The listing builds one solid part. Answer for the finished solid, in the listing's coordinates (mm). A direction names the side the tool comes from. Give positions to 0.01 mm unless a question says otherwise; leave off trailing zeros. Write each loop counter-clockwise with the first axis right and the second up, starting at its lowest first coordinate (ties: lowest second). Pieces come first, ordered by that corner, then holes.
```python
from build123d import *

# Parameters (mm, degrees)
FILLET_1_R               = 2
CHAMFER_1_SIZE           = 2
CHAMFER_2_SIZE           = 0.5
SKETCH_4_R               = 15
CUT_EXTRUDE_3_DEPTH      = 20
CHAMFER_3_SIZE           = 3
CUT_EXTRUDE_4_DEPTH      = 161.780129369
CUT_EXTRUDE_4_DEPTH_BACK = 161.780129369
SKETCH_5_R               = 5.7226
CUT_EXTRUDE_5_DEPTH      = 14.5
CUT_EXTRUDE_6_DEPTH      = 161.780129369
CUT_EXTRUDE_6_DEPTH_BACK = 161.780129369
SKETCH_7_R               = 9
SKETCH_7_R_2             = 7


with BuildPart() as part:
    # ｽｹｯﾁ1 → 回転1 (revolve)
    with BuildSketch(Plane.XY, mode=Mode.PRIVATE) as revolve_1_sk:
        Polygon((0, 0), (0, 32.5), (81, 32.5), (81, 87), (100.5, 87), (100.5, 21), (103.5, 21), (103.5, 0), align=None)
    revolve(revolve_1_sk.sketch.rotate(Axis((0, 0, 0), (1, 0, 0)), 90), axis=Axis((0, 0, 0), (1, 0, 0)))

    # ﾌｨﾚｯﾄ1
    fillet_1_edges = [part.edges().sort_by_distance(p)[0] for p in [
        (81, 0, -32.5),
    ]]
    fillet(fillet_1_edges, radius=FILLET_1_R)

    # 面取り1
    chamfer_1_edges = [part.edges().sort_by_distance(p)[0] for p in [
        (0, 0, -32.5),
    ]]
    chamfer(chamfer_1_edges, length=CHAMFER_1_SIZE)

    # 面取り2
    chamfer_2_edges = [part.edges().sort_by_distance(p)[0] for p in [
        (103.5, 0, -21),
    ]]
    chamfer(chamfer_2_edges, length=CHAMFER_2_SIZE)

    # ｽｹｯﾁ4 → ｶｯﾄ - 押し出し3 (cut)
    with BuildSketch(Plane(origin=(0, 0, 0), x_dir=(0, 0, -1), z_dir=(1, 0, 0))):
        Circle(SKETCH_4_R)
    extrude(amount=CUT_EXTRUDE_3_DEPTH, mode=Mode.SUBTRACT)

    # 面取り3
    chamfer_3_edges = [part.edges().sort_by_distance(p)[0] for p in [
        (0, 0, 15),
    ]]
    chamfer(chamfer_3_edges, length=CHAMFER_3_SIZE)

    # ｽｹｯﾁ5 → ｶｯﾄ - 押し出し4 (cut, two sides: drawn at the far end of the back side and taken through both)
    with BuildSketch(Plane(origin=(0, 0, 0), x_dir=(0, 0, -1), z_dir=(1, 0, 0)).offset(-CUT_EXTRUDE_4_DEPTH_BACK)):
        Circle(SKETCH_5_R)
    extrude(amount=CUT_EXTRUDE_4_DEPTH + CUT_EXTRUDE_4_DEPTH_BACK, mode=Mode.SUBTRACT)

    # ｽｹｯﾁ6 → ｶｯﾄ - 押し出し5 (cut)
    with BuildSketch(Plane(origin=(0, 40, 0), x_dir=(1, 0, 0), z_dir=(0, 1, 0))):
        with BuildLine():
            Line((-5, 9), (57, 9))
            ThreePointArc((57, 9), (66, 0), (57, -9))
            Line((57, -9), (-5, -9))
            ThreePointArc((-5, -9), (-14, 0), (-5, 9))
        make_face()
    extrude(amount=-CUT_EXTRUDE_5_DEPTH, mode=Mode.SUBTRACT)

    # ｽｹｯﾁ7 → ｶｯﾄ - 押し出し6 (cut, two sides: drawn at the far end of the back side and taken through both)
    with BuildSketch(Plane(origin=(0, 0, 0), x_dir=(0, 0, -1), z_dir=(1, 0, 0)).offset(-CUT_EXTRUDE_6_DEPTH_BACK)):
        with Locations((67.5, 0)):
            Circle(SKETCH_7_R)
        with Locations((33.75, 58.456714755)):
            Circle(SKETCH_7_R)
        with Locations((-33.75, 58.456714755)):
            Circle(SKETCH_7_R)
        with Locations((-67.5, 0)):
            Circle(SKETCH_7_R)
        with Locations((-33.75, -58.456714755)):
            Circle(SKETCH_7_R)
        with Locations((33.75, -58.456714755)):
            Circle(SKETCH_7_R)
        with Locations((55.858638544, 32.25)):
            Circle(SKETCH_7_R_2)
        with Locations((-55.858638544, 32.25)):
            Circle(SKETCH_7_R_2)
        with Locations((0, -64.5)):
            Circle(SKETCH_7_R_2)
    extrude(amount=CUT_EXTRUDE_6_DEPTH + CUT_EXTRUDE_6_DEPTH_BACK, mode=Mode.SUBTRACT)


solid = part.part
```
Item 1: Consider probe 1 along X at (y, z) = (40, 27); probe 2 along Y at (x, z) = (12.5, -7.5); probe 3 along X at (y, z) = (20.5, -22). Determine where each line is inside the solid, lowest interval first.
Conclusion:
probe 1: x = 81 to 100.5
probe 2: y = -31.62 to -12.99, 12.99 to 25.5
probe 3: x = 0 to 100.5
Item 2: A cutting plane is placed at D-D, the plane x = 61. Give the vertices of the cut face in (y, z), plus the area to 3 significant figures.
Conclusion:
outline: (25.5, -8.06) - (25.5, 8.06) - (31.48, 8.06) arc R32.5 ccw (long way) to (31.48, -8.06) - close; hole circle Ø11.45 at (0, 0)
area: 3,110 mm2
Item 3: Each of these flat-tipped pins is pushed along its axis until it touches: P1, Ø14.5, axis at x = 43.5, z = -3.5, coming from the +Y side; P2, Ø6, axis at x = 81, z = -36, coming from the +Y side; P3, Ø1.5, axis at y = -48.5, z = -36.5, coming from the +X side; P4, Ø11, axis at y = 32.25, z = 55.86, coming from the -X side. Where does it stop, or does it pass through?
Conclusion:
P1: stops at y = 31.23
P2: stops at y = 80.5
P3: stops at x = 100.5
P4: passes through
Item 4: A cutting plane is placed at A-A, the plane z = 0. Count the separate pieces of the cut face and the enclosed holes in it, plus the area to 3 significant figures.
Conclusion:
separate pieces: 3
enclosed holes: 0
area: 6,480 mm2
Item 5: A cutting plane is placed at C-C, the plane z = 66. Give the vertices of the cut face in (x, y), plus the area to 3 significant figures.
Conclusion:
outline: (81, -56.68) - (100.5, -56.68) - (100.5, -8.87) - (81, -8.87) - close; (81, 8.87) - (100.5, 8.87) - (100.5, 56.68) - (81, 56.68) - close
area: 1,860 mm2
Item 6: Determine the mould class of faces 1 (the face through (2.85, -9.22, 12.02)), 2 (the face through (29, 28, 9)), 3 (the face through (0.319, -30.795, 1.234)) for opening direction Y: pulls with the +Y half, pulls with the -Y half, needs draft (parallel to the pull), parting line crosses it, or undercut.
Conclusion:
face 1: undercut
face 2: needs draft
face 3: parting line crosses it
Item 7: A cutting plane is placed at B-B, the plane y = 61. Give the vertices of the cut face in (x, z), plus the area to 3 significant figures.
Conclusion:
outline: (81, -62.03) - (100.5, -62.03) - (100.5, -42.38) - (81, -42.38) - close; (81, -25.12) - (100.5, -25.12) - (100.5, 25.12) - (81, 25.12) - close; (81, 42.38) - (100.5, 42.38) - (100.5, 62.03) - (81, 62.03) - close
area: 1,750 mm2
Item 8: Which of the six approach directions +Z, -Z, +X, -X, +Y, -Y give full straight-line access (tool end or side, diameter ignored) to faces 4 (the face through (33, 25.5, 0)), 5 (the face through (100.5, 18, 18)), 6 (the face through (90.89, -86.26, -11.33)), 7 (the face through (81, 37, 1))?
Conclusion:
face 4: -X, +Y
face 5: +X
face 6: +X, -X
face 7: -X
